Source: CAD feature listing. Evaluate the final solid. Frame: model axes, mm. A direction names the side the tool comes from. Round coordinates to 2 decimals unless told otherwise and drop trailing zeros. Order: outer loops, then holes, each group sorted by start corner. A loop starts at its lowest first (then second) coordinate and runs counter-clockwise, first axis right, second up. Notation, with made-up numbers: (22, 5) -> (39, 5) arc R17 ccw to (39, 22) -> close; hole circle Ø9 at (-37.5, 24.25). An arc over 180 degrees is marked (long way). Answer as CSV lines item,"result".
Autodesk Inventor part; units mm, degrees
ref_plane "YZ Plane" through (0, 0, 0) normal (1, 0, 0) x (0, 1, 0)
ref_plane "XY Plane" through (0, 0, 0) normal (0, 0, 1) x (1, 0, 0)
sketch "Sketch1" plane through (0, 0, 0) normal (0, 0, 1) x (1, 0, 0)
  circle A0 centre (0, 0) radius 14
  circle A1 centre (0, 0) radius 16.5
  circle A2 centre (0, 0) radius 11.5
  dimension "d0" = 28
  dimension "d1" = 33
  dimension "d2" = 23
extrude "Extrusion1" add sketch "Sketch1" along normal blind 2.5 contours A0 | A1
extrude "Extrusion2" add sketch "Sketch1" against normal blind 7.5 contours A1
ref_plane "Work Plane1" through (0, -20, 0) normal (0, 1, 0) x (-1, 0, 0)
sketch "Sketch2" plane through (0, -20, 0) normal (0, 1, 0) x (-1, 0, 0)
  line L0 (-16.5, -7.5) -> (16.5, -7.5)
  line L1 (16.5, 2.5) -> (-16.5, 2.5)
  line L2 (16.5, -7.5) -> (16.5, 2.5)
  line L3 (-16.5, -7.5) -> (-16.5, 2.5)
  line L4 (-16.5, 2.5) -> (-26.5, 2.5)
  line L5 (-26.5, 2.5) -> (-26.5, -7.5)
  line L6 (-26.5, -7.5) -> (-16.5, -7.5)
  line L7 (-16.5, -7.5) -> (-16.5, 2.5)
  line L8 (16.5, 2.5) -> (26.5, 2.5)
  line L9 (26.5, 2.5) -> (26.5, -7.5)
  line L10 (26.5, -7.5) -> (16.5, -7.5)
  line L11 (16.5, -7.5) -> (16.5, 2.5)
  point P0 (0, 0)
  dimension "d8" = 10
  dimension "d9" = 10
  dimension "d10" = 10
  dimension "d11" = 10
extrude "Extrusion3" add sketch "Sketch2" along normal blind 20 contours L3 L1 L2 L0
delete faces "Delete Face1" heal yes whole lump no faces at (-3.8333, 0, -5)
extrude "Extrusion4" [suppressed]
sketch "Sketch3" plane through (0, -20, 0) normal (0, -1, 0) x (1, 0, 0)
  line L0 (-16.5, -7.5) -> (-16.5, 2.5)
  line L1 (16.5, 2.5) -> (16.5, -7.5)
  point P0 (0, 0)
  point P1 (-11.5, -2.5)
  point P2 (11.5, -2.5)
  point P3 (16.5, -2.5)
  point P4 (-16.5, -2.5)
  dimension "d23" = 5
  dimension "d24" = 5
hole "Hole1" at (-11.5, -20, -2.5) at (11.5, -20, -2.5) direction (0, 1, 0) diameter 5.35 depth 10 tip angle 118
properties part number "Adafruit_1528_4699_ND_House_02"
1. Line query: L1, parallel to Z at x = 11.5, y = -12.5 (3 decimals); L2, parallel to Y at x = -0.5, z = -3; L3, parallel to X at y = -17.5, z = -2.5 (3 decimals). Output: solid intervals per line, ascending. Write a range as [from, to].
Results below:
L1,"[-7.5, -5.175], [0.175, 2.5]"
L2,"[-20, -13.99], [13.99, 16.49]"
L3,"[-16.5, -14.175], [-8.825, 8.825], [14.175, 16.5]"
2. Pin query (flat end, axial travel): pin 1 (3 mm diameter, centred on y = 11, z = -6, fed in from +X); pin 2 (6 mm diameter, centred on y = 12.5, z = -1.5, fed in from -X); pin 3 (4.5 mm diameter, centred on x = -11.5, z = -2.5, fed in from -Y). Return the tip coordinate at first contact, or that it passes through.
Results below:
pin 1,"x = 13.49"
pin 2,"x = -13.49"
pin 3,"y = -9.74"
3. Mould query, pull axis Z, two halves, no side actions, for faces 4 (the conical face through (-12.24, -8.85, -2.33)), 5 (the flat face through (-8, -10, 2.5)), 6 (the cylindrical face through (0.363, 16.496, -2.43)), 7 (the cylindrical face through (14.11, -14.93, -1.92)). Classes: released by +Z, released by -Z, zero draft, split by the parting line, or undercut.
Results below:
face 4,"undercut"
face 5,"released by +Z"
face 6,"zero draft"
face 7,"undercut"
4. Section query C-C on y = -1. Return loops of the section in (x, z), and give its area (3 significant figures).
Results below:
outline,"(-16.5, -7.5) -> (-13.96, -7.5) -> (-13.96, 0) -> (-11.46, 0) -> (-11.46, 2.5) -> (-16.5, 2.5) -> close; (11.46, 0) -> (13.96, 0) -> (13.96, -7.5) -> (16.5, -7.5) -> (16.5, 2.5) -> (11.46, 2.5) -> close"
area,"63.3 mm2"
5. Section query A-A on y = -11. Return loops of the section in (x, z) (3 decimals), and give its area (3 significant figures).
Results below:
outline,"(-16.5, -7.5) -> (-8.66, -7.5) -> (-8.66, 0) -> (-3.354, 0) -> (-3.354, 2.5) -> (-16.5, 2.5) -> close; (3.354, 0) -> (8.66, 0) -> (8.66, -7.5) -> (16.5, -7.5) -> (16.5, 2.5) -> (3.354, 2.5) -> close; hole circle Ø5.35 at (-11.5, -2.5); hole circle Ø5.35 at (11.5, -2.5)"
area,"138 mm2"
6. Reachability of faces 1 (the cylindrical face through (-1.5, -11.4, 1.2)), 2 (the cylindrical face through (-14.15, -14.93, -2.15)), 3 (the flat face through (2, 11.5, 0)) from +Z, -Z, +X, -X, +Y, -Y: full face, straight path, thin tool, end or side. Return the list, or none.
Results below:
face 1,"+Z, -Z"
face 2,"-Y"
face 3,"-Z"
7. Section query B-B on x = 0. Return loops of the section in (y, z).
Results below:
outline,"(-20, -7.5) -> (-14, -7.5) -> (-14, 0) -> (-11.5, 0) -> (-11.5, 2.5) -> (-20, 2.5) -> close; (11.5, 0) -> (14, 0) -> (14, -7.5) -> (16.5, -7.5) -> (16.5, 2.5) -> (11.5, 2.5) -> close"
8. Section query D-D on z = 1.75. Return loops of the section in (x, y).
Results below:
outline,"(-16.5, -20) -> (16.5, -20) -> (16.5, 0) arc R16.5 ccw to (-16.5, 0) -> close; hole circle Ø23 at (0, 0)"
